Autodesk Inventor part; units mm, degrees
ref_plane "YZ Plane" through (0, 0, 0) normal (1, 0, 0) x (0, 1, 0)
ref_plane "XZ Plane" through (0, 0, 0) normal (0, 1, 0) x (-1, 0, 0)
ref_plane "XY Plane" through (0, 0, 0) normal (0, 0, 1) x (1, 0, 0)
sketch "Sketch1" plane through (0, 0, 0) normal (0, 1, 0) x (-1, 0, 0)
  line L0 (0, 0) -> (200, 0)
  line L1 (200, 0) -> (306.066, 106.066)
  line L2 (306.066, 106.066) -> (335.7645, 76.3675)
  line L3 (0, 0) -> (0, -42)
  line L4 (0, -42) -> (350, -42)
  line L5 (350, -42) -> (328.1362, 0)
  line L6 (350, -42) -> (414.721, -42) construction
  line L7 (261.897, 0) -> (328.1362, 0)
  line L8 (335.7645, 76.3675) -> (261.1647, 1.7678)
  arc A0 (261.1647, 1.7678) -> (261.897, 0) centre (259.397, 0) ccw
  line L9 (328.1362, 0) -> (328.1362, 6)
  line L10 (328.1362, 6) -> (273.8823, 6)
  line L11 (335.7645, 76.3675) -> (340.0071, 72.1249)
  line L12 (340.0071, 72.1249) -> (273.8823, 6)
  arc A1 (261.897, 0) -> (261.1647, 1.7678) centre (259.397, 0) ccw
  dimension "d0" = 200
  dimension "d1" = 150
  dimension "d2" = 135
  dimension "d3" = 42
  dimension "d4" = 42
  dimension "d5" = 350
  dimension "d6" = 117.5
  dimension "d8" = 5
  dimension "d9" = 6
  dimension "d10" = 6
  dimension "d13" = 66.2392
  dimension "d14" = 54.2539
extrude "Extrusion1" add sketch "Sketch1" along normal blind 6 contours L11 L12 L10 L9 L7 A1 L8
properties part number "A_LeftWall2(plan)_5"
Check sheet for the modelled part. Datum: model origin and axes. Units: mm. A direction names the side the tool comes from. Give positions to 0.01 mm unless a question says otherwise; leave off trailing zeros. Write each loop counter-clockwise with the first axis right and the second up, starting at its lowest first coordinate (ties: lowest second). Pieces come first, ordered by that corner, then holes. Notation, with made-up numbers: (73.5, 38.25) -> (89.5, 38.25) arc R28 cw to (89.5, 74.25) -> close; hole circle Ø3 at (-17.75, -3). An arc over 180 degrees is marked (long way). Use CSV: the item, a comma, the result in double quotes. Start each with the question number.
Q1. Release check for a two-part mould opening along Z. For faces 1 (the cylindrical face through (-261.7, 2.96, 0.97)), 2 (the flat face through (-297, 6, 30)), 3 (the flat face through (-307.41, 2.96, 39.53)) record: +Z half, -Z half, draft (parallel to the pull), parting line (faces both ways), or undercut.
Q2. Cross-section at C-C on x = -273. Enter the section's corners in (y, z).
Q3. Depth check by flat-ended pin: P1, Ø1.8, axis at x = -304.5, y = 2.5, coming from the +Z side; P2, Ø1, axis at y = 3, z = 64, coming from the -X side. Enter the tip coordinate at first touch or a pass-through.
Q4. Cross-section at B-B on y = 3.6. Enter the section's corners in (x, z), and give its area (3 significant figures).
Q5. Cross-section at D-D on z = 30.5. Enter the section's corners in (x, y), and give its area (3 significant figures).
Q6. Scan lines: line 1 along Z through (x, y) = (-314, 5.6); line 2 along Z through (x, y) = (-307, 4.45); line 3 along Z through (x, y) = (-273, 1.2). Record each from-to range of solid material in increasing order.
Q7. Cross-section at A-A on x = -321. Enter the section's corners in (y, z).
Q8. Tool access check on faces 4 (the flat face through (-295, 3, 0)), 5 (the flat face through (-301, 3, 6)), 6 (the flat face through (-328.136, 3, 3)). Record the directions out of +Z, -Z, +X, -X, +Y, -Y that give a thin tool (end or side, any length) a straight path to the whole face; none if there is none.
Working result:
1,face 1,"-Z half"
1,face 2,"draft"
1,face 3,"undercut"
2,outline,"(0, 0) -> (6, 0) -> (6, 13.6) -> (0, 13.6) -> close"
3,P1,"stops at z = 46"
3,P2,"stops at x = -332.38"
4,outline,"(-340.01, 72.12) -> (-273.88, 6) -> (-328.14, 6) -> (-328.14, 0) -> (-261.9, 0) arc R2.5 cw to (-261.16, 1.77) -> (-335.76, 76.37) -> close"
4,area,"971 mm^2"
5,outline,"(-298.38, 0) -> (-289.9, 0) -> (-289.9, 6) -> (-298.38, 6) -> close"
5,area,"50.9 mm^2"
6,line 1,"z = 0 to 6, 46.12 to 54.6"
6,line 2,"z = 0 to 6, 39.12 to 47.6"
6,line 3,"z = 0 to 13.6"
7,outline,"(0, 0) -> (6, 0) -> (6, 6) -> (0, 6) -> close; (0, 53.12) -> (6, 53.12) -> (6, 61.6) -> (0, 61.6) -> close"
8,face 4,"-Z, +X, -X, +Y, -Y"
8,face 5,"-X, +Y, -Y"
8,face 6,"-Z, -X, +Y, -Y"
